```python
from build123d import *

# Parameters (mm, degrees)
SM_BASE_FLANGE_1_DEPTH = 50
SKETCH_3_R             = 6.9
CUT_EXTRUDE_2_DEPTH    = 10
OTHER_1_DEPTH          = 71.7
CUT_EXTRUDE_3_DEPTH    = 10


# Read off the part's stored shape, not the designer's step: Затупленный угол1
# Sheet-metal steps are written as plain solids
with BuildPart() as part:
    # Sketch 1 → Базовая кромка1 (new body)
    with BuildSketch(Plane.XY):
        with BuildLine():
            Line((-351.5, 66.7), (-231.5, 66.7))
            ThreePointArc((-231.5, 66.7), (-224.428932188, 63.771067812), (-221.5, 56.7))
            Line((-221.5, 56.7), (-221.5, 15))
            ThreePointArc((-221.5, 15), (-217.106601718, 4.393398282), (-206.5, 0))
            Line((-206.5, 0), (0, 0))
            Line((0, 0), (0, 5))
            Line((0, 5), (-206.5, 5))
            ThreePointArc((-206.5, 5), (-213.571067812, 7.928932188), (-216.5, 15))
            Line((-216.5, 15), (-216.5, 56.7))
            ThreePointArc((-216.5, 56.7), (-220.893398282, 67.306601718), (-231.5, 71.7))
            Line((-231.5, 71.7), (-351.5, 71.7))
            Line((-351.5, 71.7), (-351.5, 66.7))
        make_face()
    extrude(amount=SM_BASE_FLANGE_1_DEPTH)

    # Эскиз3 → Вырез-Вытянуть2 (cut)
    with BuildSketch(Plane(origin=(0, 5, 0), x_dir=(1, 0, 0), z_dir=(0, 1, 0))):
        with Locations(Location((-17.5, -25, 0), (0, 0, 270))):
            Circle(SKETCH_3_R)
        with Locations(Location((-52.5, -25, 0), (0, 0, 270))):
            Circle(SKETCH_3_R)
    extrude(amount=-CUT_EXTRUDE_2_DEPTH, mode=Mode.SUBTRACT)

    # Other 1 outline → Other 1 (cut)
    with BuildSketch(Plane(origin=(0, 0, 0), x_dir=(1, 0, 0), z_dir=(0, 1, 0))):
        Polygon((0, 0), (-5, 0), (0, -5), align=None)
        Polygon((0, -50), (0, -45), (-5, -50), align=None)
        Polygon((-346.5, -50), (-351.5, -45), (-351.5, -50), align=None)
        Polygon((-351.5, -5), (-346.5, 0), (-351.5, 0), align=None)
    extrude(amount=OTHER_1_DEPTH, mode=Mode.SUBTRACT)

    # Эскиз4 → Вырез-Вытянуть3 (cut)
    with BuildSketch(Plane.XZ.offset(-66.7)):
        with BuildLine():
            Line((-329, 18.5), (-336, 18.5))
            ThreePointArc((-336, 18.5), (-342.5, 25), (-336, 31.5))
            Line((-336, 31.5), (-329, 31.5))
            ThreePointArc((-329, 31.5), (-322.5, 25), (-329, 18.5))
        make_face()
        with BuildLine():
            Line((-297, 18.5), (-304, 18.5))
            ThreePointArc((-304, 18.5), (-310.5, 25), (-304, 31.5))
            Line((-304, 31.5), (-297, 31.5))
            ThreePointArc((-297, 31.5), (-290.5, 25), (-297, 18.5))
        make_face()
    extrude(amount=-CUT_EXTRUDE_3_DEPTH, mode=Mode.SUBTRACT)


solid = part.part
```
Part model, mm, in its own coordinate system. A direction names the side the tool comes from. Coordinates: 2 decimals unless noted, no trailing zeros. Loops run counter-clockwise (first coordinate to the right, second up) from the corner with the lowest first, then second, coordinate; pieces in that order, holes last. Notation, with made-up numbers: (59.25, 15) - (99.25, 15) arc R11 cw to (99.25, 36) - close; hole circle Ø6 at (37.5, 23). An arc over 180 degrees is marked (long way). Write item = value, one per line. Start each with the question number.
Item 1: Flat gauge pins, fed straight in: pin 1 Ø1 at (y, z) = (44, 10) entering from -X; pin 2 Ø12 at (y, z) = (24.5, 19.5) entering from +X; pin 3 Ø5.5 at (x, y) = (-331, 69) entering from -Z; pin 4 Ø5 at (x, z) = (-259, 34) entering from -Y. Where does each tip first touch, or does it go through?
Item 2: Wall check: L1, parallel to X at y = 56, z = 3.5; L2, parallel to Z at x = -17, y = 1; L3, parallel to Y at x = -239, z = 13.5. Give the ranges that are in metal, low to high. Write a range as from..to.
Item 3: Mould opens along X. For faces 1 (the cylindrical face through (-290.5, 69.2, 25.1)), 2 (the cylindrical face through (-342.5, 69.2, 24.9)), 3 (the cylindrical face through (-213.49, 7.85, 24.65)), 4 (the flat face through (-177, 4, 0)) say: released by +X, released by -X, zero draft, split by the parting line, or undercut.
Item 4: Cut at B-B, the plane z = 10.5. Give the cut face in (x, y).
Item 5: Cut at A-A, the plane x = -17.5. Give the cut face in (y, z), and give its area (3 significant figures).
Item 6: Cut at D-D, the plane y = 30.5. Give the cut face in (x, z).
Item 7: 3-axis set-ups, long thin cutter, end or side, ignore diameter. For faces 5 (the flat face through (-292, 66.7, 19)), 6 (the flat face through (-102, 5, 25)), 7 (the cylindrical face through (-322.5, 69.2, 25.1)), 8 (the flat face through (-105, 0, 25)): which of +Z, -Z, +X, -X, +Y, -Y reach the whole face in a straight line?
Item 8: Cut at C-C, the plane z = 25. Give the cut face in (x, y).
The answers:
q1.pin_1 = -221.5
q1.pin_2 = -216.5
q1.pin_3 = 0
q1.pin_4 = 66.7
q2.L1 = -221.5..-216.5
q2.L2 = 0..18.12, 31.88..50
q2.L3 = 66.7..71.7
q3.face_1 = undercut
q3.face_2 = undercut
q3.face_3 = released by +X
q3.face_4 = zero draft
q4.outline = (-351.5, 66.7) - (-231.5, 66.7) arc R10 cw to (-221.5, 56.7) - (-221.5, 15) arc R15 ccw to (-206.5, 0) - (0, 0) - (0, 5) - (-206.5, 5) arc R10 cw to (-216.5, 15) - (-216.5, 56.7) arc R15 ccw to (-231.5, 71.7) - (-351.5, 71.7) - close
q5.outline = (0, 0) - (5, 0) - (5, 18.1) - (0, 18.1) - close; (0, 31.9) - (5, 31.9) - (5, 50) - (0, 50) - close
q5.area = 181 mm2
q6.outline = (-221.5, 0) - (-216.5, 0) - (-216.5, 50) - (-221.5, 50) - close
q7.face_5 = +Z, -Z, -X, -Y
q7.face_6 = +Z, -Z, +X, +Y
q7.face_7 = +Y, -Y
q7.face_8 = +Z, -Z, +X, -X, -Y
q8.outline = (-351.5, 66.7) - (-342.5, 66.7) - (-342.5, 71.7) - (-351.5, 71.7) - close; (-322.5, 66.7) - (-310.5, 66.7) - (-310.5, 71.7) - (-322.5, 71.7) - close; (-290.5, 66.7) - (-231.5, 66.7) arc R10 cw to (-221.5, 56.7) - (-221.5, 15) arc R15 ccw to (-206.5, 0) - (-59.4, 0) - (-59.4, 5) - (-206.5, 5) arc R10 cw to (-216.5, 15) - (-216.5, 56.7) arc R15 ccw to (-231.5, 71.7) - (-290.5, 71.7) - close; (-45.6, 0) - (-24.4, 0) - (-24.4, 5) - (-45.6, 5) - close; (-10.6, 0) - (0, 0) - (0, 5) - (-10.6, 5) - close
